Input: part model. Units: mm. Frame: model coordinates. A direction names the side the tool comes from. Coordinates: 2 decimals unless noted, no trailing zeros. Write each loop counter-clockwise with the first axis right and the second up, starting at its lowest first coordinate (ties: lowest second). Pieces come first, ordered by that corner, then holes. Notation, with made-up numbers: (75, -8.75) - (91, -8.75) arc R26 ccw to (91, 12.25) - close; hole circle Ø3 at (-33, -9). An arc over 180 degrees is marked (long way). Use CSV: the item, a comma, the result in double quotes.
```python
from build123d import *

# Parameters (mm, degrees)
SKETCH2_R          = 1.5
CUT_EXTRUDE1_DEPTH = 3.3
SKETCH3_R          = 1.5
CUT_EXTRUDE2_DEPTH = 8


with BuildPart() as part:
    # Sketch1 → Revolve1 (revolve)
    with BuildSketch(Plane.XY, mode=Mode.PRIVATE) as revolve1_sk:
        Polygon((0, 0), (0, 22.08), (-4, 22.08), (-4, 16.8), (-7, 16.8), (-7, 24), (-28, 24), (-32, 20), (-32, 2), (-44, 2), (-44, 0), align=None)
    revolve(revolve1_sk.sketch.rotate(Axis((-10, 0, 0), (1, 0, 0)), 90), axis=Axis((-10, 0, 0), (1, 0, 0)))

    # Sketch2 → Cut-Extrude1 (cut)
    with BuildSketch(Plane(origin=(0, 0, 0), x_dir=(0, 0, -1), z_dir=(1, 0, 0))):
        with Locations((-8.84, 8.84)):
            Circle(SKETCH2_R)
        with Locations((-8.84, -8.84)):
            Circle(SKETCH2_R)
        with Locations((8.84, 8.84)):
            Circle(SKETCH2_R)
        with Locations((8.84, -8.84)):
            Circle(SKETCH2_R)
    extrude(amount=-CUT_EXTRUDE1_DEPTH, mode=Mode.SUBTRACT)

    # Sketch3 → Cut-Extrude2 (cut)
    with BuildSketch(Plane(origin=(-32, 0, 0), x_dir=(0, 0, -1), z_dir=(1, 0, 0))):
        with Locations((-6, 0)):
            Circle(SKETCH3_R)
        with Locations((6, 0)):
            Circle(SKETCH3_R)
        with Locations((0, 6)):
            Circle(SKETCH3_R)
        with Locations((0, -6)):
            Circle(SKETCH3_R)
    extrude(amount=CUT_EXTRUDE2_DEPTH, mode=Mode.SUBTRACT)


solid = part.part
```
(1) Draft query along X for faces 1 (the flat face through (0, 0, 0)), 2 (the flat face through (-24, -6, 0)), 3 (the flat face through (-7, -16.3, -5)). Return one class per face: pulls with the +X half, pulls with the -X half, needs draft (parallel to the pull), parting line crosses it, or undercut.
Check values:
face 1,"pulls with the +X half"
face 2,"pulls with the -X half"
face 3,"undercut"
(2) Cut plane B-B on z = 0. Return loops of the section in (x, y), and give its area (3 significant figures).
Check values:
outline,"(-44, -2) - (-32, -2) - (-32, -4.5) - (-24, -4.5) - (-24, -7.5) - (-32, -7.5) - (-32, -20) - (-28, -24) - (-7, -24) - (-7, -16.8) - (-4, -16.8) - (-4, -22.08) - (0, -22.08) - (0, 22.08) - (-4, 22.08) - (-4, 16.8) - (-7, 16.8) - (-7, 24) - (-28, 24) - (-32, 20) - (-32, 7.5) - (-24, 7.5) - (-24, 4.5) - (-32, 4.5) - (-32, 2) - (-44, 2) - close"
area,"1,460 mm^2"
(3) Reachability of faces 4 (the cylindrical face through (-28.1, -0.9, 7.2)), 5 (the cylindrical face through (-5.521, -5.046, 16.024)), 6 (the cylindrical face through (-1.627, 10.105, -9.646)) from +Z, -Z, +X, -X, +Y, -Y: full face, straight path, thin tool, end or side. Return the list, or none.
Check values:
face 4,"-X"
face 5,"none"
face 6,"+X"
(4) Pin query (flat end, axial travel): pin 1 Ø3.5 at (y, z) = (-8.84, 8.84) entering from +X; pin 2 Ø3.5 at (y, z) = (8.84, -8.84) entering from -X; pin 3 Ø12 at (x, z) = (-23.5, -10.5) entering from -Y; pin 4 Ø10 at (x, y) = (-10.5, -9.5) entering from -Z. Return the tip coordinate at first contact, or that it passes through.
Check values:
pin 1,"x = 0"
pin 2,"x = -32"
pin 3,"y = -23.57"
pin 4,"z = -23.57"
(5) Cut plane A-A on x = -29. Return loops of the section in (y, z), and give its area (3 significant figures).
Check values:
outline,"circle Ø46 at (0, 0); hole circle Ø3 at (-6, 0); hole circle Ø3 at (0, -6); hole circle Ø3 at (0, 6); hole circle Ø3 at (6, 0)"
area,"1,630 mm^2"
(6) Ray query, probe 1 along Y at (x, z) = (-25, 0); probe 2 along X at (y, z) = (-17, 10); probe 3 along Y at (x, z) = (-1.7, 8.84). Return the intervals inside material, ascending. Write a range as from..to.
Check values:
probe 1,"-24..-7.5, -4.5..4.5, 7.5..24"
probe 2,"-32..-7, -4..0"
probe 3,"-20.23..-10.34, -7.34..7.34, 10.34..20.23"
(7) Cut plane D-D on x = -11. Return loops of the section in (y, z), and give its area (3 significant figures).
Check values:
outline,"circle Ø48 at (0, 0)"
area,"1,810 mm^2"
